For this review, use the dimensioned drawing (mm, ordinates from the lowest corner) and the shaded views. Round coordinates to 2 decimals unless told otherwise and drop trailing zeros. Write each loop counter-clockwise with the first axis right and the second up, starting at its lowest first coordinate (ties: lowest second). Pieces come first, ordered by that corner, then holes. Notation, with made-up numbers: M 17.25,45.5 L 21.25,45.5 A13 ccw 21.25,57.5 Z; hole C -23.5,53 d3. An arc over 180 degrees is marked long. Use one line per item in the form item = value. Start each with the question number.
Item 1: For line 1 (X direction, y = 1.25, z = 19.05); line 2 (Z direction, x = 6.35, y = 1.2); line 3 (Z direction, x = 5, y = 1.5), list the stretches that pass through material, from the lowest coordinate up. Write a range as [from, to].
Item 2: Draft analysis for pull direction Z (two halves, no side actions). For the marked faces 1, 2, 3 and 4, state which applies: released by +Z, released by -Z, zero draft, split by the parting line, or undercut.
Item 3: For P1, Ø1, axis at x = 4.5, z = 20.5, coming from the +Y side, flat-tipped, find the tip position at first contact; note if it passes through.
Item 4: Add section D-D (y = 2.3). State the section outline as (x, z) points (3 decimals), and give its area (3 significant figures).
Item 5: Add section A-A (z = 19.05). State the section outline as (x, y) points (3 decimals).
Item 6: Add section B-B (x = 6.35). State the section outline as (y, z) points (3 decimals), and give its area (3 significant figures).
Item 7: Add section C-C (y = 0.75). State the section outline as (x, z) points.
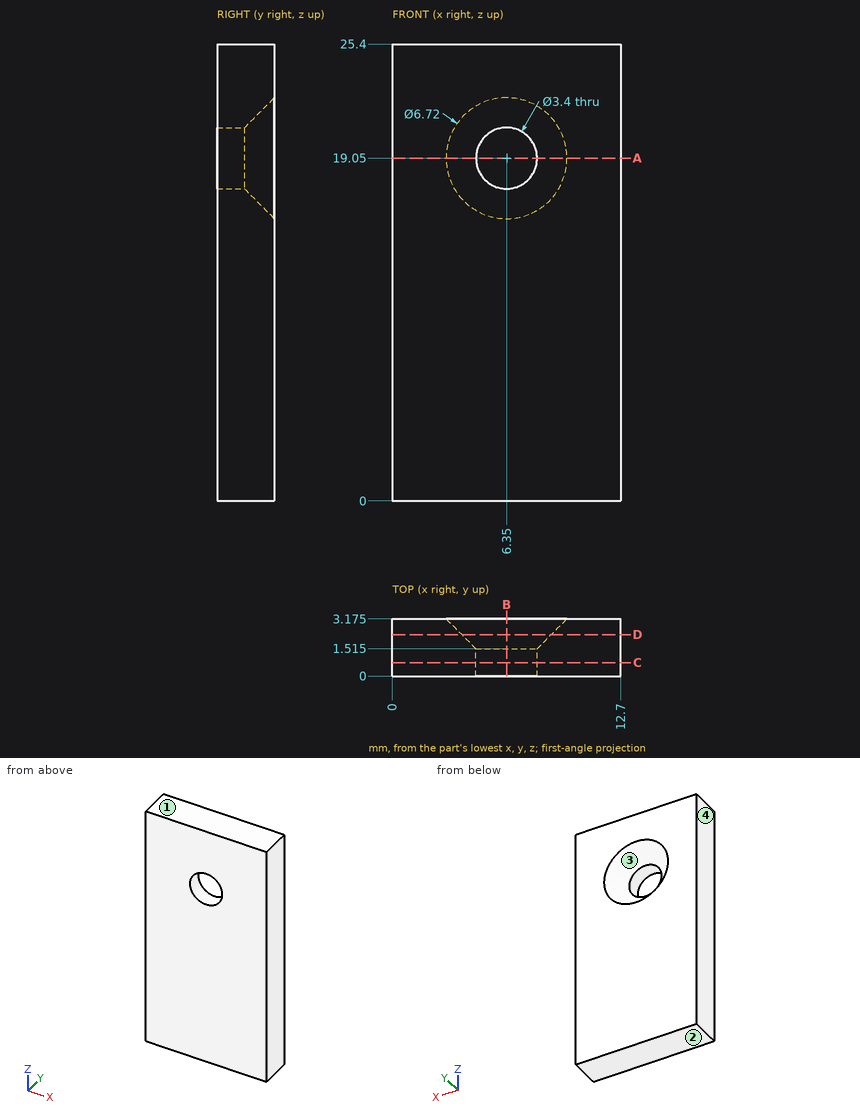
Calculated:
q1.line_1 = [0, 4.65], [8.05, 12.7]
q1.line_2 = [0, 17.35], [20.75, 25.4]
q1.line_3 = [0, 18.02], [20.08, 25.4]
q2.face_1 = released by +Z
q2.face_2 = released by -Z
q2.face_3 = undercut
q2.face_4 = zero draft
q3.P1 = 2.67
q4.outline = M 0,0 L 12.7,0 L 12.7,25.4 L 0,25.4 Z; hole C 6.35,19.05 d4.97
q4.area = 303 mm^2
q5.outline = M 0,0 L 4.65,0 L 4.65,1.515 L 2.99,3.175 L 0,3.175 Z; M 8.05,0 L 12.7,0 L 12.7,3.175 L 9.71,3.175 L 8.05,1.515 Z
q6.outline = M 0,0 L 3.175,0 L 3.175,15.69 L 1.515,17.35 L 0,17.35 Z; M 0,20.75 L 1.515,20.75 L 3.175,22.41 L 3.175,25.4 L 0,25.4 Z
q6.area = 67.1 mm^2
q7.outline = M 0,0 L 12.7,0 L 12.7,25.4 L 0,25.4 Z; hole C 6.35,19.05 d3.4
